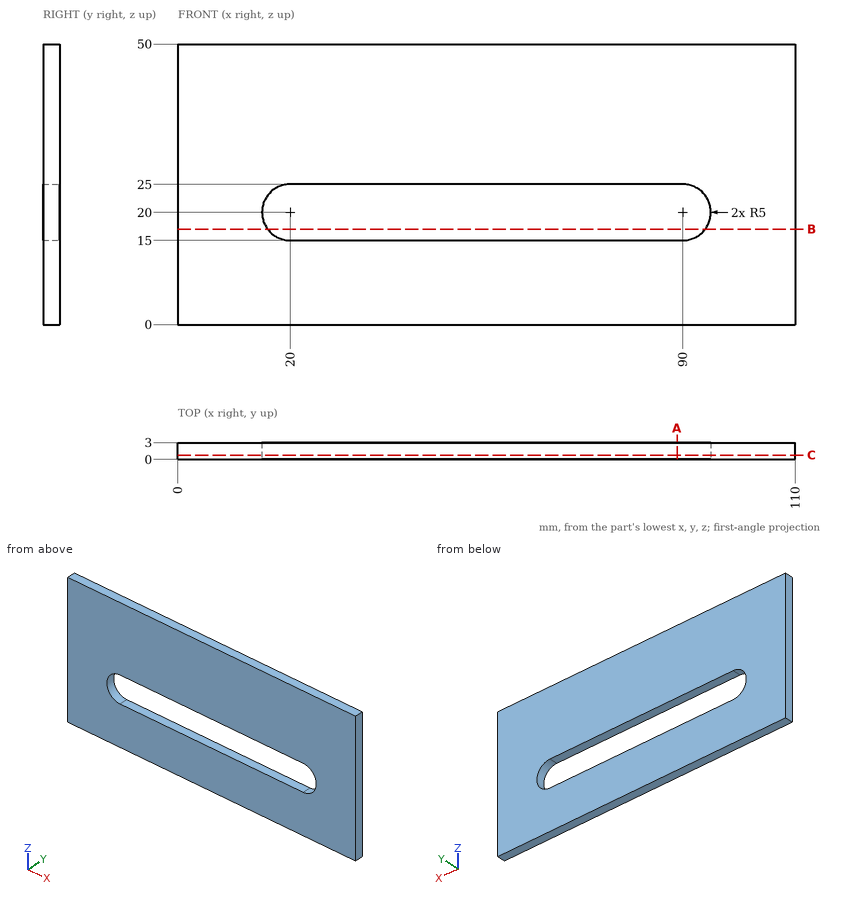
Answer from the drawing. Dimensions are ordinates in mm from the lowest x, y and z of the part. Coordinates: 2 decimals unless noted, no trailing zeros. Order: outer loops, then holes, each group sorted by start corner. A loop starts at its lowest first (then second) coordinate and runs counter-clockwise, first axis right, second up. Notation, with made-up numbers: (89.25, -32) -> (106.25, -32) arc R12 ccw to (106.25, -23) -> close; hole circle Ø10 at (-5.75, 43). An arc over 180 degrees is marked (long way). Answer as a JSON object with one key per item and string values.
1) A cutting plane is placed at C-C, the plane y = 0.75. Determine the outline of the cut face in (x, z), plus the area to 3 significant figures.
Model answer:
{"outline": "(0, 0) -> (110, 0) -> (110, 50) -> (0, 50) -> close; hole (20, 15) -> (90, 15) arc R5 ccw to (90, 25) -> (20, 25) arc R5 ccw to start", "area": "4,720 mm²"}
2) Consider line 1 along Z through (x, y) = (31, 0.45); line 2 along X through (y, z) = (1.9, 24); line 3 along Z through (x, y) = (16, 1.7). Determine where each line is inside the solid, lowest interval first. Write a range as from..to.
Model answer:
{"line 1": "z = 0..15, 25..50", "line 2": "x = 0..17, 93..110", "line 3": "z = 0..17, 23..50"}
3) A cutting plane is placed at A-A, the plane x = 89. Determine the outline of the cut face in (y, z).
Model answer:
{"outline": "(0, 0) -> (3, 0) -> (3, 15) -> (0, 15) -> close; (0, 25) -> (3, 25) -> (3, 50) -> (0, 50) -> close"}
4) This flat-tipped pin is pushed along its axis until it touches: pin 1 (2 mm diameter, centred on x = 79.5, z = 7, fed in from -Y). Where does it stop, or does it pass through?
Model answer:
{"pin 1": "stops at y = 0"}
5) A cutting plane is placed at B-B, the plane z = 17. Determine the outline of the cut face in (x, y), plus the area to 3 significant figures.
Model answer:
{"outline": "(0, 0) -> (16, 0) -> (16, 3) -> (0, 3) -> close; (94, 0) -> (110, 0) -> (110, 3) -> (94, 3) -> close", "area": "96.0 mm²"}
